Verification items for this drawing (mm, ordinates from the low corner). A direction names the side the tool comes from. Round coordinates to 2 decimals unless told otherwise and drop trailing zeros. Loops run counter-clockwise (first coordinate to the right, second up) from the corner with the lowest first, then second, coordinate; pieces in that order, holes last. Notation, with made-up numbers: M -40,10 L 15,10 A35 cw 15,42 Z; hole C -36,14.5 d3. An arc over 180 degrees is marked long. Answer in a Markdown table with one row per item. Add a question column.
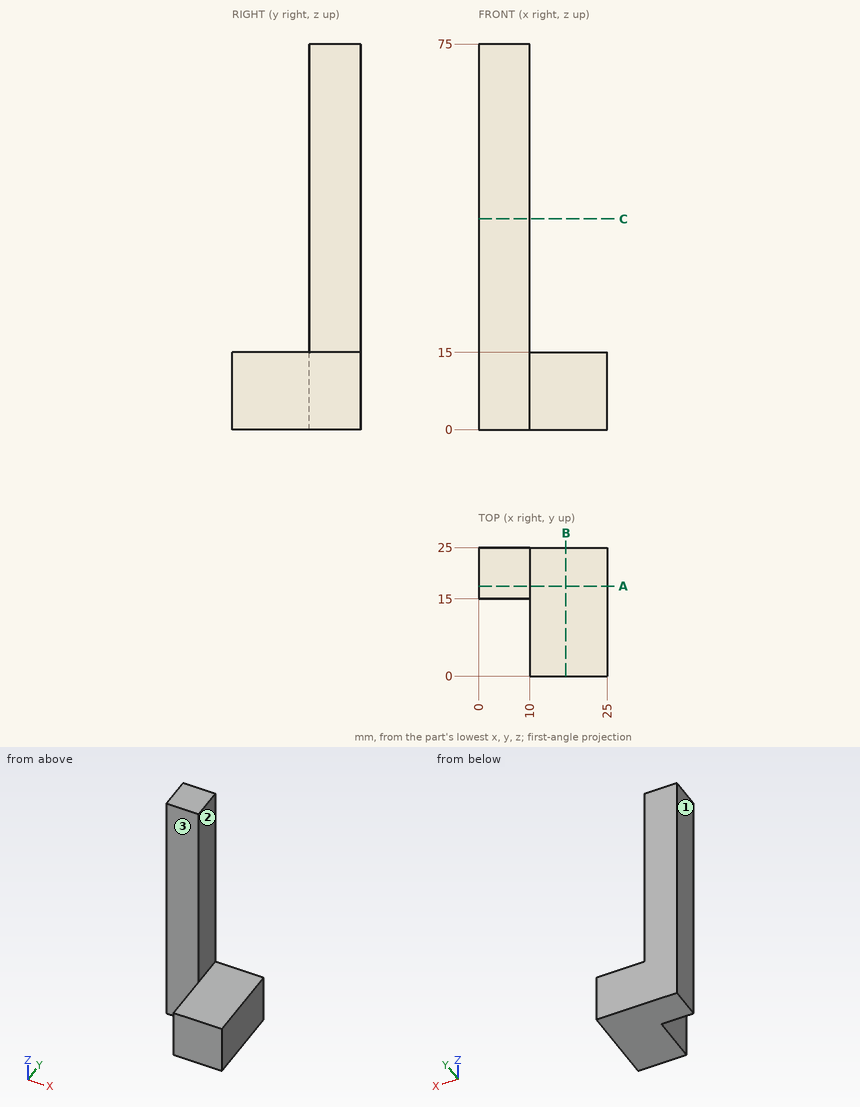
1) Cross-section at B-B, the plane x = 17. Record the boundary of the cut face in (y, z).
2) Cross-section at C-C, the plane z = 41. Record the boundary of the cut face in (x, y), plus the area to 3 significant figures.
3) Thickness scan on L1, parallel to X at y = 17, z = 42; L2, parallel to Z at x = 13, y = 4.25; L3, parallel to Y at x = 1.75, z = 4. Record the ranges inside material, lowest first. Write a range as [from, to].
4) Go/stop test with flat-tipped pins: pin 1 (1.5 mm diameter, centred on x = 7.5, y = 13.5, fed in from +Z); pin 2 (12 mm diameter, centred on x = 17, y = 14.5, fed in from +Z); pin 3 (12 mm diameter, centred on y = 19.5, z = 30, fed in from -X); pin 4 (8 mm diameter, centred on y = 21.5, z = 59, fed in from +X). Record where each tip stops, or that it passes through.
5) Cross-section at A-A, the plane y = 17.5. Record the boundary of the cut face in (x, z), plus the area to 3 significant figures.
6) Set-up check for the marked faces 1, 2 and 3: record each of +Z, -Z, +X, -X, +Y, -Y from which the full face is reachable in a straight line by a thin tool's end or side.
Worked answers:
| question | item | result |
|---|---|---|
| 1 | outline | M 0,0 L 25,0 L 25,15 L 0,15 Z |
| 2 | outline | M 0,15 L 10,15 L 10,25 L 0,25 Z |
| 2 | area | 100 mm2 |
| 3 | L1 | x = [0, 10] |
| 3 | L2 | z = [0, 15] |
| 3 | L3 | y = [15, 25] |
| 4 | pin 1 | passes through |
| 4 | pin 2 | stops at z = 15 |
| 4 | pin 3 | stops at x = 0 |
| 4 | pin 4 | stops at x = 10 |
| 5 | outline | M 0,0 L 25,0 L 25,15 L 10,15 L 10,75 L 0,75 Z |
| 5 | area | 975 mm2 |
| 6 | face 1 | +Z, -Z, -X, +Y, -Y |
| 6 | face 2 | +Z, +X, +Y, -Y |
| 6 | face 3 | +Z, -Z, -X, -Y |
